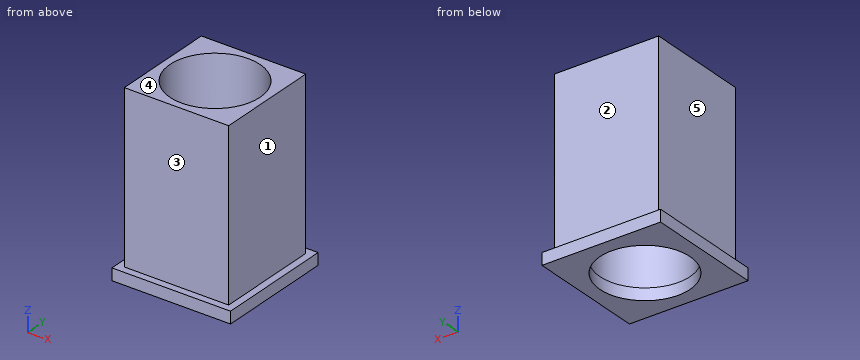
from build123d import *

# Parameters (mm, degrees)
F0_W      = 50
F0_H      = 50
F1_DEPTH  = 5
F2_W      = 44
F2_H      = 44
F2_R      = 19
F3_DEPTH  = 70
F3_FACE_R = 19
F4_DEPTH  = 78.5


with BuildPart() as f1:
    # F0 (on Top) → F1 (new body)
    with BuildSketch(Plane.XY):
        Rectangle(F0_W, F0_H)
    extrude(amount=F1_DEPTH)

    # F2 (on face) → F3 (join)
    with BuildSketch(Plane.XY.offset(5)):
        Rectangle(F2_W, F2_H)
        Circle(F2_R, mode=Mode.SUBTRACT)
    extrude(amount=F3_DEPTH)

    # F3_face (on face) → F4 (cut)
    with BuildSketch(Plane.XY.offset(5)):
        Circle(F3_FACE_R)
    extrude(amount=-F4_DEPTH, mode=Mode.SUBTRACT)


solid = f1.part
Input: part model. Units: mm. Frame: model coordinates. Face numbers are marked on the shaded views. A direction names the side the tool comes from. Round coordinates to 2 decimals unless told otherwise and drop trailing zeros. Order: outer loops, then holes, each group sorted by start corner. A loop starts at its lowest first (then second) coordinate and runs counter-clockwise, first axis right, second up. Notation, with made-up numbers: (-25.5, 64) - (17.5, 64) arc R9 ccw to (17.5, 73) - close; hole circle Ø1 at (-38.75, 47). An arc over 180 degrees is marked (long way). Use a Markdown table: item, result.
1. First-contact query: pin 1 (1.5 mm diameter, centred on y = -2.5, z = 39.5, fed in from +X); pin 2 (4 mm diameter, centred on x = -16, y = 3, fed in from +Z); pin 3 (3 mm diameter, centred on y = 4.5, z = 9, fed in from -X); pin 4 (13 mm diameter, centred on x = 3.5, z = 45, fed in from -Y). Flat tips, straight axial feed; report the tip coordinate or a pass-through.
Evaluation:
| item | result |
|---|---|
| pin 1 | x = 22 |
| pin 2 | through |
| pin 3 | x = -22 |
| pin 4 | y = -22 |
2. Section A-A on y = 0. Return the cut outline in (x, z).
Evaluation:
| item | result |
|---|---|
| outline | (-25, 0) - (-19, 0) - (-19, 75) - (-22, 75) - (-22, 5) - (-25, 5) - close; (19, 0) - (25, 0) - (25, 5) - (22, 5) - (22, 75) - (19, 75) - close |
3. Section C-C on y = 21. Return the cut outline in (x, z), then the cut area to 3 significant figures.
Evaluation:
| item | result |
|---|---|
| outline | (-25, 0) - (25, 0) - (25, 5) - (22, 5) - (22, 75) - (-22, 75) - (-22, 5) - (-25, 5) - close |
| area | 3,330 mm^2 |
4. Section D-D on z = 37.5. Return the cut outline in (x, y).
Evaluation:
| item | result |
|---|---|
| outline | (-22, -22) - (22, -22) - (22, 22) - (-22, 22) - close; hole circle Ø38 at (0, 0) |
5. Access query for the marked faces 1, 2, 3, 4 and 5. Directions: +Z, -Z, +X, -X, +Y, -Y. A direction counts if a zero-diameter tool reaches every point of the face in a straight line with its end or side. Return the directions, or none.
Evaluation:
| item | result |
|---|---|
| face 1 | +Z, +X, +Y, -Y |
| face 2 | +Z, +X, -X, +Y |
| face 3 | +Z, +X, -X, -Y |
| face 4 | +Z, +X, -X, +Y, -Y |
| face 5 | +Z, -X, +Y, -Y |
6. Material intervals for probe 1 along Y at (x, z) = (0, 3); probe 2 along Y at (x, z) = (0, 21); probe 3 along Z at (x, y) = (23, -9.5), sorted ascending.
Evaluation:
| item | result |
|---|---|
| probe 1 | -25 to -19, 19 to 25 |
| probe 2 | -22 to -19, 19 to 22 |
| probe 3 | 0 to 5 |
